from build123d import *

# Parameters (mm, degrees)
SKETCH1_R                                           = 14
BOSS_EXTRUDE1_DEPTH                                 = 4
SKETCH2_R                                           = 8.5
CUT_EXTRUDE1_DEPTH                                  = 21.199009877
SKETCH3_R                                           = 11
BOSS_EXTRUDE2_DEPTH                                 = 28
SKETCH4_R                                           = 10
CUT_EXTRUDE2_DEPTH                                  = 28
BOSS_EXTRUDE3_START                                 = -12
BOSS_EXTRUDE3_DEPTH                                 = 12
BOSS_EXTRUDE4_DEPTH                                 = 9
BOSS_EXTRUDE4_DEPTH_BACK                            = 9
CUT_EXTRUDE7_START                                  = -19
CUT_EXTRUDE7_DEPTH                                  = 19
CUT_EXTRUDE8_REACH                                  = 48.701
CUT_EXTRUDE8_END_RADIUS                             = 10
SKETCH8_W                                           = 1
SKETCH8_H                                           = 21.539335767
CUT_EXTRUDE9_START                                  = -4
SKETCH9_R                                           = 8.5
CUT_EXTRUDE9_DEPTH                                  = 4
CHAMFER1_SIZE                                       = 1.3
CHAMFER2_SIZE                                       = 0.8
CHAMFER4_SIZE                                       = 0.2
CHAMFER5_SIZE                                       = 0.2
CHAMFER6_SIZE                                       = 3.464101615
CHAMFER6_SIZE_2                                     = 2
CUT_EXTRUDE10_DEPTH                                 = 39.845849199
CUT_EXTRUDE10_DEPTH_BACK                            = 39.845849199
CUT_EXTRUDE12_DEPTH                                 = 39.845849281
CUT_EXTRUDE12_DEPTH_BACK                            = 39.845849281
SKETCH11_R                                          = 2.5
CSK_FOR_M3_COUNTERSUNK_FLAT_HEAD_SCREW1_D           = 3
CSK_FOR_M3_COUNTERSUNK_FLAT_HEAD_SCREW1_DEPTH       = 5
CSK_FOR_M3_COUNTERSUNK_FLAT_HEAD_SCREW1_CSINK_D     = 4
CSK_FOR_M3_COUNTERSUNK_FLAT_HEAD_SCREW1_CSINK_ANGLE = 90
CSK_FOR_M3_COUNTERSUNK_FLAT_HEAD_SCREW1_TIP         = 0.901290929
CUT_EXTRUDE13_DEPTH                                 = 39.845849281
CUT_EXTRUDE13_DEPTH_BACK                            = 39.845849281
SKETCH15_R                                          = 1.5
SKETCH16_R                                          = 2.5
CUT_EXTRUDE14_DEPTH                                 = 6.6


# Read off the part's stored shape, not the designer's step: Cut-Extrude7
with BuildPart() as part:
    # Sketch1 → Boss-Extrude1 (new body)
    with BuildSketch(Plane.XY):
        Circle(SKETCH1_R)
    extrude(amount=BOSS_EXTRUDE1_DEPTH)

    # Sketch2 → Cut-Extrude1 (cut, through all)
    with BuildSketch(Plane(origin=(0, 0, 0), x_dir=(-1, 0, 0), z_dir=(0, 0, -1))):
        Circle(SKETCH2_R)
    extrude(amount=-CUT_EXTRUDE1_DEPTH, mode=Mode.SUBTRACT)

    # Sketch3 → Boss-Extrude2 (add)
    with BuildSketch(Plane.XY.offset(4)):
        Circle(SKETCH3_R)
    extrude(amount=BOSS_EXTRUDE2_DEPTH)

    # Sketch4 → Cut-Extrude2 (cut)
    with BuildSketch(Plane.XY.offset(32)):
        Circle(SKETCH4_R)
    extrude(amount=-CUT_EXTRUDE2_DEPTH, mode=Mode.SUBTRACT)

    # Sketch5 → Boss-Extrude3 (add)
    with BuildSketch(Plane.XY.offset(32).offset(BOSS_EXTRUDE3_START)):
        with BuildLine():
            Line((3.158488565, 17), (-3.158488565, 17))
            Line((-3.158488565, 17), (-9.622511389, 5.329847518))
            ThreePointArc((-9.622511389, 5.329847518), (0, 11), (9.622511389, 5.329847518))
            Line((9.622511389, 5.329847518), (3.158488565, 17))
        make_face()
    extrude(amount=BOSS_EXTRUDE3_DEPTH)

    # Sketch6 → Boss-Extrude4 (add, two sides: drawn at the far end of the back side and taken through both)
    with BuildSketch(Plane(origin=(0, 0, 0), x_dir=(0, 0, -1), z_dir=(1, 0, 0)).offset(-BOSS_EXTRUDE4_DEPTH_BACK)):
        with BuildLine():
            Line((0, 9.5), (0, -9.5))
            Line((0, -9.5), (11, -9.5))
            ThreePointArc((11, -9.5), (12.414213562, -8.914213562), (13, -7.5))
            Line((13, -7.5), (13, -3.7))
            ThreePointArc((13, -3.7), (13.058578644, -3.558578644), (13.2, -3.5))
            Line((13.2, -3.5), (19.6, -3.5))
            ThreePointArc((19.6, -3.5), (19.882842712, -3.382842712), (20, -3.1))
            Line((20, -3.1), (20, -2.5))
            ThreePointArc((20, -2.5), (16.485281374, 5.985281374), (8, 9.5))
            Line((8, 9.5), (0, 9.5))
        make_face()
    extrude(amount=BOSS_EXTRUDE4_DEPTH + BOSS_EXTRUDE4_DEPTH_BACK)

    # Cut-Extrude7 outline → Cut-Extrude7 (cut)
    with BuildSketch(Plane(origin=(0, 9.5, 0), x_dir=(1, 0, 0), z_dir=(0, 1, 0)).offset(CUT_EXTRUDE7_START)):
        with BuildLine():
            ThreePointArc((-4, 4.0001), (0, 0.0001), (4, 4.0001))
            Line((4, 4.0001), (4, 20))
            Line((4, 20), (-4, 20))
            Line((-4, 20), (-4, 4.0001))
        make_face()
    extrude(amount=CUT_EXTRUDE7_DEPTH, mode=Mode.SUBTRACT)

    # Cut-Extrude8: up to this cylinder (the profile starts outside it)
    cut_extrude8_end = Plane(origin=(0, 0, 21.230332), z_dir=(0, 0, 1)) * Cylinder(CUT_EXTRUDE8_END_RADIUS, 118.402, mode=Mode.PRIVATE)
    # Sketch8 → Cut-Extrude8 (cut, up to the surface)
    with BuildSketch(Plane(origin=(0, 17, 0), x_dir=(1, 0, 0), z_dir=(0, 1, 0)), mode=Mode.PRIVATE) as cut_extrude8_sk1:
        with Locations((0, -21.230332117)):
            Rectangle(SKETCH8_W, SKETCH8_H)
    cut_extrude8_tool1 = extrude(cut_extrude8_sk1.sketch, amount=-CUT_EXTRUDE8_REACH, mode=Mode.PRIVATE) - cut_extrude8_end
    add(cut_extrude8_tool1.solids().sort_by_distance((0, 17, 21.230332))[0], mode=Mode.SUBTRACT)

    # Sketch9 → Cut-Extrude9 (cut)
    with BuildSketch(Plane.XY.offset(CUT_EXTRUDE9_START)):
        with Locations(Location((0, 0, 0), (0, 0, 180))):
            Circle(SKETCH9_R)
    extrude(amount=CUT_EXTRUDE9_DEPTH, mode=Mode.SUBTRACT)

    # Chamfer1
    chamfer1_edges = [part.edges().sort_by_distance(p)[0] for p in [
        (-14, 0, 4),
    ]]
    chamfer(chamfer1_edges, length=CHAMFER1_SIZE)

    # Chamfer2
    chamfer2_edges = [part.edges().sort_by_distance(p)[0] for p in [
        (-14, 0, 0),
    ]]
    chamfer(chamfer2_edges, length=CHAMFER2_SIZE)

    # Chamfer4
    chamfer4_edges = [part.edges().sort_by_distance(p)[0] for p in [
        (9, -3.382842712, -19.882842712),
        (-9, -3.5, -16.4),
        (9, -3.558578644, -13.058578644),
        (-9, -5.6, -13),
        (9, -8.914213562, -12.414213562),
        (-9, -9.5, -5.5),
        (-9, 9.5, -4),
        (-9, 5.985281374, -16.485281374),
        (-9, -2.8, -20),
        (-9, -3.382842712, -19.882842712),
        (-9, -3.558578644, -13.058578644),
        (-9, -8.914213562, -12.414213562),
        (9, -2.8, -20),
        (9, 5.985281374, -16.485281374),
        (9, 9.5, -4),
        (9, -9.5, -5.5),
        (9, -5.6, -13),
        (9, -3.5, -16.4),
    ]]
    chamfer(chamfer4_edges, length=CHAMFER4_SIZE)

    # Chamfer5
    chamfer5_edges = [part.edges().sort_by_distance(p)[0] for p in [
        (-1.829244283, 17, 20),
        (-1.829244283, 17, 32),
        (1.829244283, 17, 20),
        (1.829244283, 17, 32),
    ]]
    chamfer(chamfer5_edges, length=CHAMFER5_SIZE)

    # Chamfer6
    # the kernel refuses this chamfer: 3.464101615, 2 mm, written as the material it takes off along each edge
    with BuildSketch(Plane(origin=(0, 0, 10.460664233), x_dir=(-0.757967837141711, 0.6522919268691869, 0), z_dir=(-0.6522919268691869, -0.757967837141711, 0))) as chamfer6_piece_1_section:
        Polygon((11, CHAMFER6_SIZE), (11 - CHAMFER6_SIZE_2, 0), (11, 0), align=None)
    chamfer6_piece_1 = revolve(axis=Axis((0, 0, 10.460664233), (0, 0, -1)), revolution_arc=98.570745894, mode=Mode.PRIVATE)
    chamfer6_piece_1 = split(chamfer6_piece_1, bisect_by=Plane(origin=(-0.5, 10.551597033, 9.113518596), z_dir=(1, 0, 0)), keep=Keep.TOP, mode=Mode.PRIVATE)
    chamfer6_piece_1 = split(chamfer6_piece_1, bisect_by=Plane(origin=(0.5, 10.551597033, 9.113518596), z_dir=(-1, 0, 0)), keep=Keep.TOP, mode=Mode.PRIVATE)
    add(chamfer6_piece_1, mode=Mode.SUBTRACT)

    # Sketch10 → Cut-Extrude10 (cut, two sides: drawn at the far end of the back side and taken through both)
    with BuildSketch(Plane(origin=(0, 0, 0), x_dir=(0, 0, -1), z_dir=(1, 0, 0)).offset(-CUT_EXTRUDE10_DEPTH_BACK)):
        with BuildLine():
            Line((-25.5, 1.5), (-7.5, 1.5))
            ThreePointArc((-7.5, 1.5), (-6, 0), (-7.5, -1.5))
            Line((-7.5, -1.5), (-25.5, -1.5))
            ThreePointArc((-25.5, -1.5), (-27, 0), (-25.5, 1.5))
        make_face()
    extrude(amount=CUT_EXTRUDE10_DEPTH + CUT_EXTRUDE10_DEPTH_BACK, mode=Mode.SUBTRACT)

    # Sketch11 → Cut-Extrude12 (cut, two sides: drawn at the far end of the back side and taken through both)
    with BuildSketch(Plane(origin=(0, 0, 0), x_dir=(0, 0, -1), z_dir=(1, 0, 0)).offset(-CUT_EXTRUDE12_DEPTH_BACK)):
        with Locations((6.50011, 2)):
            Circle(SKETCH11_R)
    extrude(amount=CUT_EXTRUDE12_DEPTH + CUT_EXTRUDE12_DEPTH_BACK, mode=Mode.SUBTRACT)

    # CSK for M3 Countersunk Flat Head Screw1
    with Locations(Plane.ZY.offset(9)):
        with Locations((-6.50011, -6), (-15.50011, 2)):
            CounterSinkHole(CSK_FOR_M3_COUNTERSUNK_FLAT_HEAD_SCREW1_D / 2, CSK_FOR_M3_COUNTERSUNK_FLAT_HEAD_SCREW1_CSINK_D / 2, depth=CSK_FOR_M3_COUNTERSUNK_FLAT_HEAD_SCREW1_DEPTH, counter_sink_angle=CSK_FOR_M3_COUNTERSUNK_FLAT_HEAD_SCREW1_CSINK_ANGLE)
            with Locations((0, 0, -(CSK_FOR_M3_COUNTERSUNK_FLAT_HEAD_SCREW1_DEPTH + CSK_FOR_M3_COUNTERSUNK_FLAT_HEAD_SCREW1_TIP / 2))):  # 118° drill point
                Cone(0, CSK_FOR_M3_COUNTERSUNK_FLAT_HEAD_SCREW1_D / 2, CSK_FOR_M3_COUNTERSUNK_FLAT_HEAD_SCREW1_TIP, mode=Mode.SUBTRACT)

    # Sketch15 → Cut-Extrude13 (cut, two sides: drawn at the far end of the back side and taken through both)
    with BuildSketch(Plane(origin=(0, 0, 0), x_dir=(0, 0, -1), z_dir=(1, 0, 0)).offset(-CUT_EXTRUDE13_DEPTH_BACK)):
        with Locations(Location((-29.45, 13.994315244, 0), (0, 0, 90))):
            Circle(SKETCH15_R)
        with Locations(Location((-23.7, 13.994315244, 0), (0, 0, 90))):
            Circle(SKETCH15_R)
    extrude(amount=CUT_EXTRUDE13_DEPTH + CUT_EXTRUDE13_DEPTH_BACK, mode=Mode.SUBTRACT)

    # Sketch16 → Cut-Extrude14 (cut)
    with BuildSketch(Plane(origin=(10, 0, 0), x_dir=(0, 0, -1), z_dir=(1, 0, 0))):
        with Locations((-29.45, 13.994315244)):
            Circle(SKETCH16_R)
        with Locations((-23.7, 13.994315244)):
            Circle(SKETCH16_R)
    extrude(amount=-CUT_EXTRUDE14_DEPTH, mode=Mode.SUBTRACT)


solid = part.part
Design review of the part built by this model. Coordinates are the model's own, in mm. A direction names the side the tool comes from. Round coordinates to 2 decimals unless told otherwise and drop trailing zeros. Write each loop counter-clockwise with the first axis right and the second up, starting at its lowest first coordinate (ties: lowest second). Pieces come first, ordered by that corner, then holes.
Item 1: For faces 4 (the flat face through (-6, -6, -13)), 5 (the flat face through (1, -10, 0)), 6 (the cylindrical face through (-10.5, 0, 6)), 7 (the flat face through (-4.5, -7.4, 4)), list the 3-axis set-ups (+Z, -Z, +X, -X, +Y, -Y) from which the entire face can be reached by the end or side of a thin tool; tool diameter is ignored.
Item 2: Consider section A-A on z = 28.5. Give the boundary of the cut face in (x, y), and give its area (3 significant figures).
Item 3: For pin 1 Ø2.5 at (y, z) = (13.99, 29.45) entering from +X; pin 2 Ø12 at (x, z) = (-0.5, 3) entering from +Y; pin 3 Ø4 at (x, y) = (7, -5) entering from -Z; pin 4 Ø1.5 at (x, y) = (8.5, 3) entering from +Z, all flat-tipped, find the tip position at first contact; note any pin that passes through.
Item 4: Wall thickness on L1, parallel to X at y = -1.5, z = 26; L2, parallel to Y at x = 1.3, z = 23.7; L3, parallel to Z at x = -6.8, y = -6: over which ranges is each line inside the solid? List them lowest first.
Item 5: Consider section B-B on x = 2.5. Count the separate pieces of the cut face and the enclosed holes in it, and give its area (3 significant figures).
Item 6: Draft analysis for pull direction Y (two halves, no side actions). For faces 1 (the flat face through (-9, 0, -10)), 2 (the flat face through (-4.03, -9.5, -2.98)), 3 (the cylindrical face through (9.54, 3, 18.2)), state which applies: released by +Y, released by -Y, zero draft, split by the parting line, or undercut.
Check values:
1. face 4: -Z, +X, -X, -Y
1. face 5: -Z
1. face 6: +X, -X
1. face 7: +Z
2. outline: (-9.62, 5.33) arc R11 ccw (long way) to (9.62, 5.33) - (6.1, 11.68) - (3.4, 11.68) - (3.4, 12.83) - (0.5, 12.83) - (0.5, 9.99) arc R10 cw (long way) to (-0.5, 9.99) - (-0.5, 12.83) - (-5.47, 12.83) - close; (-4.18, 15.16) - (-0.5, 15.16) - (-0.5, 17) - (-3.16, 17) - close; (0.5, 15.16) - (3.4, 15.16) - (3.4, 16.31) - (3.54, 16.31) - (3.16, 17) - (0.5, 17) - close
2. area: 107 mm2
3. pin 1: passes through
3. pin 2: stops at y = 14
3. pin 3: stops at z = -20
3. pin 4: stops at z = 4
4. L1: x = -10.9 to -9.89, 9.89 to 10.9
4. L2: y = -10.92 to -9.92, 9.92 to 12.49, 15.49 to 17
4. L3: z = -13 to -8, -5 to 4
5. separate pieces: 2
5. enclosed holes: 2
5. area: 164 mm2
6. face 1: zero draft
6. face 2: released by -Y
6. face 3: undercut
